Work out the finished part from the listing and answer in its coordinate system (mm). Round coordinates to 2 decimals unless told otherwise and drop trailing zeros. Order: outer loops, then holes, each group sorted by start corner. A loop starts at its lowest first (then second) coordinate and runs counter-clockwise, first axis right, second up. Notation, with made-up numbers: (-16.5, 25.25) - (6.5, 25.25) arc R23 cw to (6.5, 62.25) - close; hole circle Ø2 at (57, 23). An arc over 180 degrees is marked (long way). Use one line per item in the form item = value. Start each with the question number.
Q1. Find the intervals of material crossed by line 1 (Y direction, x = 76, z = 966.5); line 2 (Y direction, x = 63, z = 386.5), in increasing order. Write a range as [from, to].
Q2. The part is cut by section B-B on y = -88.5. Determine the outline of the cut face in (x, z), plus the area to 3 significant figures.
Q3. The part is cut by section A-A on z = 865. Determine the outline of the cut face in (x, y).
Q4. Given P1, Ø6, axis at x = -63, z = 505.5, coming from the +Y side; P2, Ø2, axis at x = 57.5, z = 681.5, coming from the -Y side, each flat-ended and moving along its own axis, determine where each tip first touches the part or whether it passes through.
from build123d import *

# Parameters (mm, degrees)
SKETCH1_W           = 200
SKETCH1_H           = 250
BOSS_EXTRUDE1_DEPTH = 1100
FILLET1_R           = 50
FILLET2_R           = 50
FILLET3_R           = 50
FILLET4_R           = 50


with BuildPart() as part:
    # Sketch1 → Boss-Extrude1 (new body)
    with BuildSketch(Plane.XY):
        Rectangle(SKETCH1_W, SKETCH1_H)
    extrude(amount=BOSS_EXTRUDE1_DEPTH)

    # Fillet1
    fillet1_edges = [part.edges().sort_by_distance(p)[0] for p in [
        (-100, 125, 550),
    ]]
    fillet(fillet1_edges, radius=FILLET1_R)

    # Fillet2
    fillet2_edges = [part.edges().sort_by_distance(p)[0] for p in [
        (-100, -125, 550),
    ]]
    fillet(fillet2_edges, radius=FILLET2_R)

    # Fillet3
    fillet3_edges = [part.edges().sort_by_distance(p)[0] for p in [
        (100, 125, 550),
    ]]
    fillet(fillet3_edges, radius=FILLET3_R)

    # Fillet4
    fillet4_edges = [part.edges().sort_by_distance(p)[0] for p in [
        (100, -125, 550),
    ]]
    fillet(fillet4_edges, radius=FILLET4_R)


solid = part.part
Found:
q1.line_1 = [-117.71, 117.71]
q1.line_2 = [-123.28, 123.28]
q2.outline = (-98.14, 0) - (98.14, 0) - (98.14, 1100) - (-98.14, 1100) - close
q2.area = 216,000 mm²
q3.outline = (-100, -75) arc R50 ccw to (-50, -125) - (50, -125) arc R50 ccw to (100, -75) - (100, 75) arc R50 ccw to (50, 125) - (-50, 125) arc R50 ccw to (-100, 75) - close
q4.P1 = 123.99
q4.P2 = -124.58
